For this review, take the finished solid that the model builds, in its own axes (mm). A direction names the side the tool comes from. Round coordinates to 2 decimals unless told otherwise and drop trailing zeros. Write each loop counter-clockwise with the first axis right and the second up, starting at its lowest first coordinate (ties: lowest second). Pieces come first, ordered by that corner, then holes. Notation, with made-up numbers: M 81.5,3.25 L 117.5,3.25 A13 ccw 117.5,13.25 Z; hole C 24,32.25 d7. An arc over 180 degrees is marked long. One line per question, with ' | ' between items.
```python
from build123d import *

# Parameters (mm, degrees)
SKETCH1_W           = 12
SKETCH1_H           = 24
BOSS_EXTRUDE1_DEPTH = 5.5
SKETCH2_W           = 2
SKETCH2_H           = 24
BOSS_EXTRUDE2_DEPTH = 29.5
BOSS_EXTRUDE4_START = 3
SKETCH4_W           = 5.5
SKETCH4_H           = 24
BOSS_EXTRUDE4_DEPTH = 18
SKETCH5_W           = 9.25
SKETCH5_H           = 18
CUT_EXTRUDE1_DEPTH  = 1.5
FILLET1_R           = 2.5
SKETCH6_R           = 2.25
CUT_EXTRUDE2_DEPTH  = 31.170349683
FILLET2_R           = 1.5


with BuildPart() as part:
    # Sketch1 → Boss-Extrude1 (new body)
    with BuildSketch(Plane(origin=(0, 0, 0), x_dir=(1, 0, 0), z_dir=(0, 1, 0))):
        Rectangle(SKETCH1_W, SKETCH1_H)
    extrude(amount=BOSS_EXTRUDE1_DEPTH)

    # Sketch2 → Boss-Extrude2 (add)
    with BuildSketch(Plane(origin=(0, 0, 0), x_dir=(1, 0, 0), z_dir=(0, 1, 0))):
        with Locations((7, 0)):
            Rectangle(SKETCH2_W, SKETCH2_H)
    extrude(amount=BOSS_EXTRUDE2_DEPTH)

    # Sketch4 → Boss-Extrude4 (add)
    with BuildSketch(Plane(origin=(0, 5.5, 0), x_dir=(1, 0, 0), z_dir=(0, 1, 0)).offset(BOSS_EXTRUDE4_START)):
        with Locations((3.25, 0)):
            Rectangle(SKETCH4_W, SKETCH4_H)
    extrude(amount=BOSS_EXTRUDE4_DEPTH)

    # Sketch5 → Cut-Extrude1 (cut)
    with BuildSketch(Plane.ZY.offset(-0.5)):
        with Locations((0, 17.5)):
            Rectangle(SKETCH5_W, SKETCH5_H)
    extrude(amount=-CUT_EXTRUDE1_DEPTH, mode=Mode.SUBTRACT)

    # Fillet1
    # the kernel refuses this fillet: 2.5 mm, written as the material it takes off along each edge
    with BuildSketch(Plane(origin=(0.5, 32.228219619, 4.625), x_dir=(0, 0, 1), z_dir=(0, -1, 0)), Plane(origin=(0.5, 8.5, -4.625), x_dir=(0, 0, -1), z_dir=(0, 1, 0))) as fillet1_piece_1:
        with BuildLine():
            CenterArc((2.291287847, -2.5), FILLET1_R, 90, 66.421821522)
            Line((0, -1.5), (0, 0))
            Line((0, 0), (2.291287847, 0))
        make_face()
    extrude(amount=23.728219619, mode=Mode.SUBTRACT)

    # Sketch6 → Cut-Extrude2 (cut, through all)
    with BuildSketch(Plane(origin=(0, 26.5, 0), x_dir=(1, 0, 0), z_dir=(0, 1, 0))):
        with Locations(Location((3, -6, 0), (0, 0, 270))):
            Circle(SKETCH6_R)
        with Locations(Location((3, 6, 0), (0, 0, 270))):
            Circle(SKETCH6_R)
    extrude(amount=-CUT_EXTRUDE2_DEPTH, mode=Mode.SUBTRACT)

    # Fillet2
    fillet2_edges = [part.edges().sort_by_distance(p)[0] for p in [
        (0.5, 17.5, -12),
        (0.5, 17.5, 12),
    ]]
    fillet(fillet2_edges, radius=FILLET2_R)


solid = part.part
```
Item 1: Machinability: for faces 1 (the face through (2, 18, 0)), 2 (the face through (0.5, 17, 9)), 3 (the face through (4, 8.5, 0)), which of the approach directions +Z, -Z, +X, -X, +Y, -Y give a long, thin tool a straight path to every point of the face, cutting with its end or side? Answer none if there is none.
Results:
face 1: -X, +Y | face 2: +Z, -Z, -X, +Y | face 3: +Z, -Z, -X
Item 2: Insertion check: pin 1 Ø2.5 at (y, z) = (19, -1) entering from -X; pin 2 Ø5 at (y, z) = (16, 6.5) entering from -X; pin 3 Ø5 at (x, z) = (3, -6) entering from +Y; pin 4 Ø1.5 at (x, y) = (3, 6.5) entering from -Z. Each pin has a flat end and moves straight along its axis. Give the tip position at first contact, or say it passes through.
Results:
pin 1: x = 2 | pin 2: x = 0.5 | pin 3: y = 26.5 | pin 4: through
Item 3: Take a section at A-A (x = 4.25). Write out the cut boundary in (y, z).
Results:
outline: M 0,-12 L 5.5,-12 L 5.5,-7.87 L 0,-7.87 Z; M 0,-4.13 L 5.5,-4.13 L 5.5,4.13 L 0,4.13 Z; M 0,7.87 L 5.5,7.87 L 5.5,12 L 0,12 Z; M 8.5,-12 L 26.5,-12 L 26.5,-7.87 L 8.5,-7.87 Z; M 8.5,-4.13 L 26.5,-4.13 L 26.5,4.13 L 8.5,4.13 Z; M 8.5,7.87 L 26.5,7.87 L 26.5,12 L 8.5,12 Z
Item 4: Take a section at C-C (y = 10.5). Write out the cut boundary in (x, z), then the cut area to 3 significant figures.
Results:
outline: M 0.5,-10.5 A1.5 ccw 2,-12 L 8,-12 L 8,12 L 2,12 A1.5 ccw 0.5,10.5 L 0.5,6.92 A2.5 ccw 0.76,5.81 A2.25 cw long 2,3.98 L 2,-3.98 A2.25 cw long 0.76,-5.81 A2.5 ccw 0.5,-6.92 Z | area: 133 mm2
Item 5: To check wall thickness, follow line 1 along Y through (x, z) = (5.25, -10.25); line 2 along Z through (x, y) = (3, 18.5); line 3 along X through (y, z) = (2.5, -6). State the ranges of each line that lie inside material, in increasing order. Write a range as from..to.
Results:
line 1: 0..5.5, 8.5..26.5 | line 2: -12..-8.25, -3.75..3.75, 8.25..12 | line 3: -6..0.75, 5.25..8
Item 6: Mouldability with a two-part tool opening along Z and no side actions: class faces 4 (the face through (4.813, 17.626, 7.333)), 5 (the face through (2.5, 11.3, -12)), 6 (the face through (0.5, 17, -9)) as +Z half, -Z half, draft (parallel to the pull), parting line (faces both ways), or undercut.
Results:
face 4: undercut | face 5: -Z half | face 6: draft
Item 7: Take a section at D-D (z = -5). Write out the cut boundary in (x, y).
Results:
outline: M -6,0 L 0.98,0 L 0.98,5.5 L -6,5.5 Z; M 5.02,0 L 8,0 L 8,29.5 L 6,29.5 L 6,26.5 L 5.02,26.5 L 5.02,8.5 L 6,8.5 L 6,5.5 L 5.02,5.5 Z
Item 8: Take a section at B-B (z = -2.25). Write out the cut boundary in (x, y), then the cut area to 3 significant figures.
Results:
outline: M -6,0 L 8,0 L 8,29.5 L 6,29.5 L 6,26.5 L 2,26.5 L 2,8.5 L 6,8.5 L 6,5.5 L -6,5.5 Z | area: 197 mm2
